Geometry: see drawing. Coordinates: mm, zero at the bounding-box minimum. A direction names the side the tool comes from. Give positions to 0.01 mm unless a question says otherwise; leave off trailing zeros. Loops run counter-clockwise (first coordinate to the right, second up) from the corner with the lowest first, then second, coordinate; pieces in that order, holes last. Notation, with made-up numbers: M 57,89.25 L 87,89.25 A31 cw 87,117.25 Z; hole C -17.75,18.25 d2. An arc over 180 degrees is marked long. Put each result on its own line as item: value.
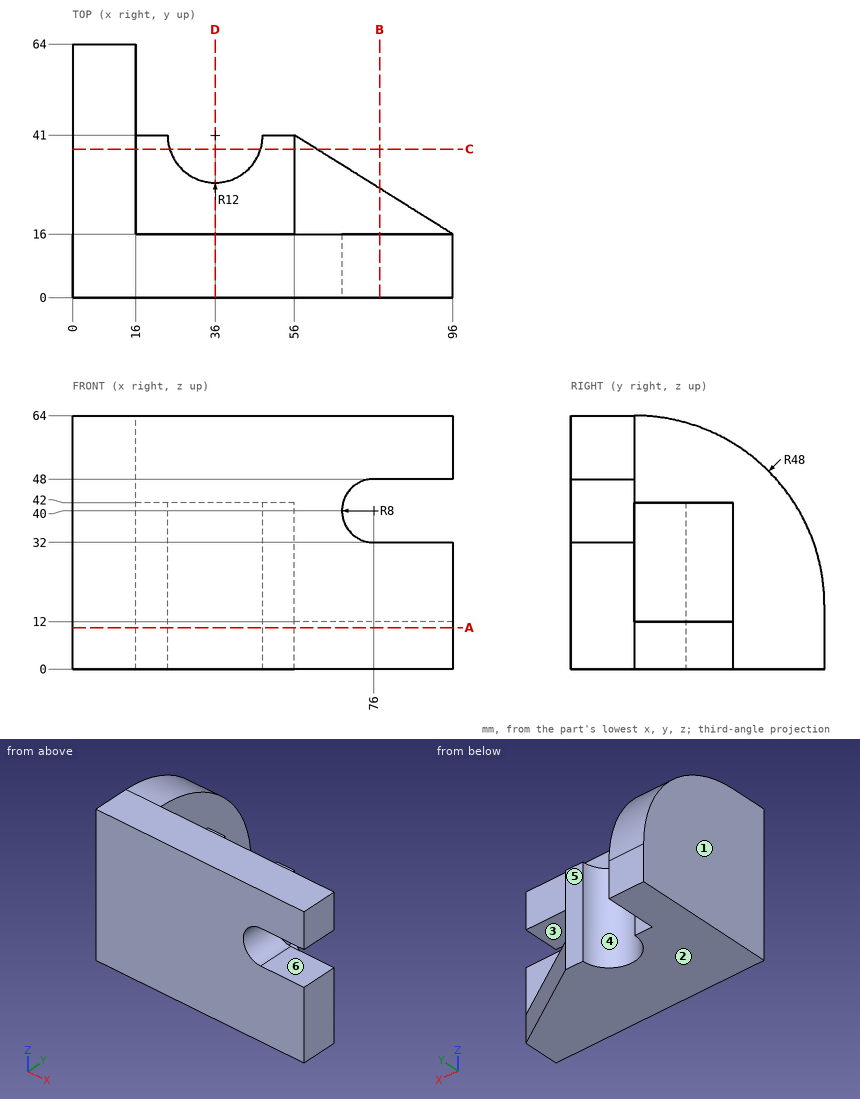
Item 1: Section A-A on z = 10.5. Output: boundary loops of the cut face in (x, y), then the cut area to 3 significant figures.
Output values:
outline: M 0,0 L 96,0 L 96,16 L 56,41 L 48,41 A12 cw 24,41 L 16,41 L 16,64 L 0,64 Z
area: 3,580 mm²
Item 2: Line query: probe 1 along X at (y, z) = (47, 19); probe 2 along X at (y, z) = (19, 37.5). Output: solid intervals per line, ascending. Write a range as [from, to].
Output values:
probe 1: [0, 16]
probe 2: [0, 56]
Item 3: Section B-B on x = 77.5. Output: boundary loops of the cut face in (y, z).
Output values:
outline: M 0,0 L 27.56,0 L 27.56,12 L 16,12 L 16,32 L 0,32 Z; M 0,48 L 16,48 L 16,64 L 0,64 Z
Item 4: Mould query, pull axis Z, two halves, no side actions, for the marked faces 1, 2 and 3. Classes: pulls with the +Z half, pulls with the -Z half, needs draft (parallel to the pull), parting line crosses it, or undercut.
Output values:
face 1: needs draft
face 2: pulls with the -Z half
face 3: undercut
Item 5: Pin query (flat end, axial travel): pin 1 Ø7.5 at (y, z) = (31.5, 22.5) entering from +X; pin 2 Ø4 at (x, z) = (11.5, 40) entering from +Y; pin 3 Ø4 at (x, z) = (53, 12.5) entering from +Y. Return the tip coordinate at first contact, or that it passes through.
Output values:
pin 1: x = 56
pin 2: y = 58.66
pin 3: y = 41
Item 6: Section D-D on x = 36. Output: boundary loops of the cut face in (y, z), then the cut area to 3 significant figures.
Output values:
outline: M 0,0 L 29,0 L 29,42 L 16,42 L 16,64 L 0,64 Z
area: 1,570 mm²
Item 7: Set-up query: the marked faces 4, 5 and 6. Return all of +Z, -Z, +X, -X, +Y, -Y with unobstructed straight access to the full face (end or side cutting, diameter ignored); none if empty.
Output values:
face 4: +Z, -Z, +Y
face 5: +Z, -Z, +X, +Y
face 6: +X, +Y, -Y
Item 8: Section C-C on y = 37.5. Output: boundary loops of the cut face in (x, z).
Output values:
outline: M 0,0 L 24.52,0 L 24.52,42 L 16,42 L 16,58.92 L 0,58.92 Z; M 47.48,0 L 61.6,0 L 61.6,12 L 56,12 L 56,42 L 47.48,42 Z
